from build123d import *

# Parameters (mm, degrees)
BOSS_EXTRUDE1_DEPTH = 120
SKETCH3_W           = 120
SKETCH3_H           = 10
BOSS_EXTRUDE2_DEPTH = 50
SKETCH11_R          = 13
CUT_EXTRUDE3_DEPTH  = 120
SKETCH7_R           = 1.825
SKETCH7_R_2         = 2
CUT_EXTRUDE6_DEPTH  = 5
CUT_EXTRUDE12_DEPTH = 4
SKETCH10_R          = 13
CUT_EXTRUDE13_DEPTH = 116
SKETCH8_R           = 1.825
SKETCH8_R_2         = 2
CUT_EXTRUDE14_DEPTH = 5
SKETCH13_R          = 13
CUT_EXTRUDE17_DEPTH = 120
SKETCH17_R          = 13
CUT_EXTRUDE18_DEPTH = 6
SKETCH18_R          = 1.75
CUT_EXTRUDE19_DEPTH = 6
FILLET1_R           = 3
FILLET2_R           = 3
CHAMFER1_SIZE       = 3
SKETCH19_W          = 15
SKETCH19_H          = 15
CUT_EXTRUDE20_DEPTH = 115
SKETCH20_R          = 5
CUT_EXTRUDE21_DEPTH = 5
FILLET3_R           = 3
SKETCH21_W          = 15
SKETCH21_H          = 15
CUT_EXTRUDE22_DEPTH = 5
SKETCH22_R          = 5
CUT_EXTRUDE23_DEPTH = 5
FILLET4_R           = 3
CUT_EXTRUDE24_START = -5
SKETCH23_R          = 1.825
SKETCH23_R_2        = 2
CUT_EXTRUDE24_DEPTH = 5
CUT_EXTRUDE25_START = -5
SKETCH24_R          = 1.825
SKETCH24_R_2        = 2
CUT_EXTRUDE25_DEPTH = 5
SKETCH26_R          = 1.825
SKETCH26_R_2        = 2
CUT_EXTRUDE26_DEPTH = 5


with BuildPart() as part:
    # Sketch1 → Boss-Extrude1 (new body)
    with BuildSketch(Plane(origin=(0, 0, 0), x_dir=(1, 0, 0), z_dir=(0, 1, 0))):
        Polygon((-60, 60), (-60, -60), (60, -60), (60, 60), (0, 60), align=None)
    extrude(amount=BOSS_EXTRUDE1_DEPTH)

    # Sketch3 → Boss-Extrude2 (add)
    with BuildSketch(Plane(origin=(60, 0, 0), x_dir=(0, 0, -1), z_dir=(1, 0, 0))):
        with Locations((0, 5)):
            Rectangle(SKETCH3_W, SKETCH3_H)
    extrude(amount=BOSS_EXTRUDE2_DEPTH)

    # Sketch11 → Cut-Extrude3 (cut)
    with BuildSketch(Plane.XY.offset(60)):
        with Locations((0, 60)):
            Circle(SKETCH11_R)
    extrude(amount=-CUT_EXTRUDE3_DEPTH, mode=Mode.SUBTRACT)

    # Sketch7 → Cut-Extrude6 (cut)
    with BuildSketch(Plane.ZY.offset(60)):
        with Locations((0, 76)):
            Circle(SKETCH7_R)
        with Locations((13.856406461, 52)):
            Circle(SKETCH7_R)
        with Locations((-13.856406461, 52)):
            Circle(SKETCH7_R)
        with Locations((-38.183766184, 98.183766184)):
            Circle(SKETCH7_R_2)
        with Locations((38.183766184, 98.183766184)):
            Circle(SKETCH7_R_2)
        with Locations((38.183766184, 21.816233816)):
            Circle(SKETCH7_R_2)
        with Locations((-38.183766184, 21.816233816)):
            Circle(SKETCH7_R_2)
    extrude(amount=-CUT_EXTRUDE6_DEPTH, mode=Mode.SUBTRACT)

    # Sketch4 → Cut-Extrude12 (cut)
    with BuildSketch(Plane.XZ):
        Polygon((16, 16), (110, 16), (110, -16), (16, -16), (16, -60), (-16, -60), (-16, -16), (-60, -16), (-60, 16), (-16, 16), (-16, 60), (16, 60), align=None)
    extrude(amount=-CUT_EXTRUDE12_DEPTH, mode=Mode.SUBTRACT)

    # Sketch10 → Cut-Extrude13 (cut)
    with BuildSketch(Plane(origin=(0, 120, 0), x_dir=(1, 0, 0), z_dir=(0, 1, 0))):
        with Locations(Location((0, 0, 0), (0, 0, 270))):
            Circle(SKETCH10_R)
    extrude(amount=-CUT_EXTRUDE13_DEPTH, mode=Mode.SUBTRACT)

    # Sketch8 → Cut-Extrude14 (cut)
    with BuildSketch(Plane(origin=(0, 0, -60), x_dir=(-1, 0, 0), z_dir=(0, 0, -1))):
        with Locations((0, 76)):
            Circle(SKETCH8_R)
        with Locations((13.856406461, 52)):
            Circle(SKETCH8_R)
        with Locations((-13.856406461, 52)):
            Circle(SKETCH8_R)
        with Locations((-38.183766184, 98.183766184)):
            Circle(SKETCH8_R_2)
        with Locations((38.183766184, 98.183766184)):
            Circle(SKETCH8_R_2)
        with Locations((38.183766184, 21.816233816)):
            Circle(SKETCH8_R_2)
        with Locations((-38.183766184, 21.816233816)):
            Circle(SKETCH8_R_2)
    extrude(amount=-CUT_EXTRUDE14_DEPTH, mode=Mode.SUBTRACT)

    # Sketch13 → Cut-Extrude17 (cut)
    with BuildSketch(Plane(origin=(60, 0, 0), x_dir=(0, 0, -1), z_dir=(1, 0, 0))):
        with Locations((0, 60)):
            Circle(SKETCH13_R)
    extrude(amount=-CUT_EXTRUDE17_DEPTH, mode=Mode.SUBTRACT)

    # Sketch17 → Cut-Extrude18 (cut)
    with BuildSketch(Plane(origin=(0, 10, 0), x_dir=(1, 0, 0), z_dir=(0, 1, 0))):
        with Locations(Location((85, 0, 0), (0, 0, 270))):
            Circle(SKETCH17_R)
    extrude(amount=-CUT_EXTRUDE18_DEPTH, mode=Mode.SUBTRACT)

    # Sketch18 → Cut-Extrude19 (cut)
    with BuildSketch(Plane(origin=(0, 10, 0), x_dir=(1, 0, 0), z_dir=(0, 1, 0))):
        with Locations(Location((93, 13.856406461, 0), (0, 0, 270))):
            Circle(SKETCH18_R)
        with Locations(Location((69, 0, 0), (0, 0, 270))):
            Circle(SKETCH18_R)
        with Locations(Location((93, -13.856406461, 0), (0, 0, 270))):
            Circle(SKETCH18_R)
    extrude(amount=-CUT_EXTRUDE19_DEPTH, mode=Mode.SUBTRACT)

    # Fillet1
    fillet1_edges = [part.edges().sort_by_distance(p)[0] for p in [
        (16, 2, -16),
        (-16, 2, -16),
        (-16, 2, 16),
        (16, 2, 16),
    ]]
    fillet(fillet1_edges, radius=FILLET1_R)

    # Fillet2
    fillet2_edges = [part.edges().sort_by_distance(p)[0] for p in [
        (0, 4, -13),
    ]]
    fillet(fillet2_edges, radius=FILLET2_R)

    # Chamfer1
    chamfer1_edges = [part.edges().sort_by_distance(p)[0] for p in [
        (0, 4, 60),
        (110, 4, 0),
        (0, 4, -60),
        (-60, 4, 0),
    ]]
    chamfer(chamfer1_edges, length=CHAMFER1_SIZE)

    # Sketch19 → Cut-Extrude20 (cut)
    with BuildSketch(Plane(origin=(0, 120, 0), x_dir=(1, 0, 0), z_dir=(0, 1, 0))):
        with Locations((-52.5, 52.5)):
            Rectangle(SKETCH19_W, SKETCH19_H)
        with Locations((-52.5, -52.5)):
            Rectangle(SKETCH19_W, SKETCH19_H)
    extrude(amount=-CUT_EXTRUDE20_DEPTH, mode=Mode.SUBTRACT)

    # Sketch20 → Cut-Extrude21 (cut)
    with BuildSketch(Plane(origin=(0, 5, 0), x_dir=(1, 0, 0), z_dir=(0, 1, 0))):
        with Locations(Location((-52.5, 52.5, 0), (0, 0, 270))):
            Circle(SKETCH20_R)
        with Locations(Location((-52.5, -52.5, 0), (0, 0, 270))):
            Circle(SKETCH20_R)
    extrude(amount=-CUT_EXTRUDE21_DEPTH, mode=Mode.SUBTRACT)

    # Fillet3
    fillet3_edges = [part.edges().sort_by_distance(p)[0] for p in [
        (-45, 62.5, -45),
        (-45, 62.5, 45),
    ]]
    fillet(fillet3_edges, radius=FILLET3_R)

    # Sketch21 → Cut-Extrude22 (cut)
    with BuildSketch(Plane(origin=(0, 10, 0), x_dir=(1, 0, 0), z_dir=(0, 1, 0))):
        with Locations((102.5, -52.5)):
            Rectangle(SKETCH21_W, SKETCH21_H)
        with Locations((102.5, 52.5)):
            Rectangle(SKETCH21_W, SKETCH21_H)
    extrude(amount=-CUT_EXTRUDE22_DEPTH, mode=Mode.SUBTRACT)

    # Sketch22 → Cut-Extrude23 (cut)
    with BuildSketch(Plane(origin=(0, 5, 0), x_dir=(1, 0, 0), z_dir=(0, 1, 0))):
        with Locations(Location((102.5, 52.5, 0), (0, 0, 270))):
            Circle(SKETCH22_R)
        with Locations(Location((102.5, -52.5, 0), (0, 0, 270))):
            Circle(SKETCH22_R)
    extrude(amount=-CUT_EXTRUDE23_DEPTH, mode=Mode.SUBTRACT)

    # Fillet4
    fillet4_edges = [part.edges().sort_by_distance(p)[0] for p in [
        (95, 7.5, 45),
        (95, 7.5, -45),
    ]]
    fillet(fillet4_edges, radius=FILLET4_R)

    # Sketch23 → Cut-Extrude24 (cut)
    with BuildSketch(Plane.XY.offset(60).offset(CUT_EXTRUDE24_START)):
        with Locations((0.077859326, 75.922140674)):
            Circle(SKETCH23_R)
        with Locations((13.934265787, 51.922140674)):
            Circle(SKETCH23_R)
        with Locations((-13.778547134, 51.922140674)):
            Circle(SKETCH23_R)
        with Locations(Location((-38.183766184, 98.183766184, 0), (0, 0, 180))):
            Circle(SKETCH23_R_2)
        with Locations(Location((38.183766184, 98.183766184, 0), (0, 0, 180))):
            Circle(SKETCH23_R_2)
        with Locations(Location((38.183766184, 21.816233816, 0), (0, 0, 180))):
            Circle(SKETCH23_R_2)
        with Locations(Location((-38.183766184, 21.816233816, 0), (0, 0, 180))):
            Circle(SKETCH23_R_2)
    extrude(amount=CUT_EXTRUDE24_DEPTH, mode=Mode.SUBTRACT)

    # Sketch24 → Cut-Extrude25 (cut)
    with BuildSketch(Plane(origin=(60, 0, 0), x_dir=(0, 0, -1), z_dir=(1, 0, 0)).offset(CUT_EXTRUDE25_START)):
        with Locations(Location((0, 76, 0), (0, 0, 180))):
            Circle(SKETCH24_R)
        with Locations(Location((13.856406461, 52, 0), (0, 0, 180))):
            Circle(SKETCH24_R)
        with Locations(Location((-13.856406461, 52, 0), (0, 0, 180))):
            Circle(SKETCH24_R)
        with Locations(Location((-38.183766184, 98.183766184, 0), (0, 0, 180))):
            Circle(SKETCH24_R_2)
        with Locations(Location((38.183766184, 98.183766184, 0), (0, 0, 180))):
            Circle(SKETCH24_R_2)
        with Locations(Location((38.183766184, 21.816233816, 0), (0, 0, 180))):
            Circle(SKETCH24_R_2)
        with Locations(Location((-38.183766184, 21.816233816, 0), (0, 0, 180))):
            Circle(SKETCH24_R_2)
    extrude(amount=CUT_EXTRUDE25_DEPTH, mode=Mode.SUBTRACT)

    # Sketch26 → Cut-Extrude26 (cut)
    with BuildSketch(Plane(origin=(0, 120, 0), x_dir=(1, 0, 0), z_dir=(0, 1, 0))):
        with Locations(Location((0, 16, 0), (0, 0, 270))):
            Circle(SKETCH26_R)
        with Locations(Location((13.856406461, -8, 0), (0, 0, 270))):
            Circle(SKETCH26_R)
        with Locations(Location((-13.856406461, -8, 0), (0, 0, 270))):
            Circle(SKETCH26_R)
        with Locations(Location((-38.183766184, 38.183766184, 0), (0, 0, 270))):
            Circle(SKETCH26_R_2)
        with Locations(Location((38.183766184, 38.183766184, 0), (0, 0, 270))):
            Circle(SKETCH26_R_2)
        with Locations(Location((38.183766184, -38.183766184, 0), (0, 0, 270))):
            Circle(SKETCH26_R_2)
        with Locations(Location((-38.183766184, -38.183766184, 0), (0, 0, 270))):
            Circle(SKETCH26_R_2)
    extrude(amount=-CUT_EXTRUDE26_DEPTH, mode=Mode.SUBTRACT)


solid = part.part
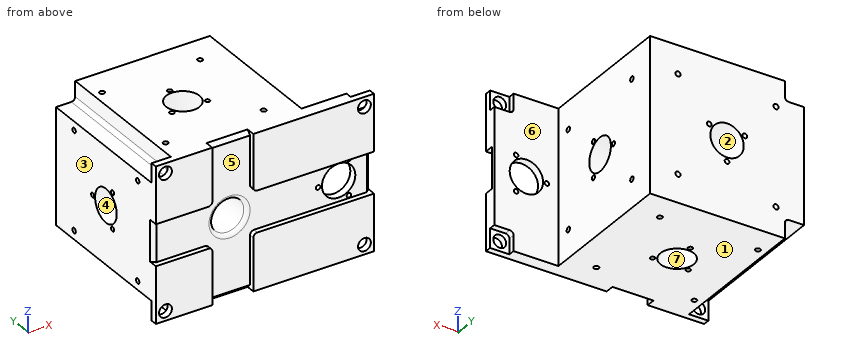
Build history of the part. All positions in model axes, mm. Face numbers are marked on the shaded views. A direction names the side the tool comes from. Round coordinates to 2 decimals unless told otherwise and drop trailing zeros. Write each loop counter-clockwise with the first axis right and the second up, starting at its lowest first coordinate (ties: lowest second). Pieces come first, ordered by that corner, then holes. Notation, with made-up numbers: M 30,84.5 L 39,84.5 A16 ccw 39,110.5 Z; hole C 78,30.5 d11. An arc over 180 degrees is marked long. Use CSV: the item, a comma, the result in double quotes.
1. Two-plate mould, pull along Z, no slides. Class the marked faces 1, 2, 3 and 4: +Z half, -Z half, draft (parallel to the pull), parting line (faces both ways), or undercut.
Reply:
face 1,"-Z half"
face 2,"undercut"
face 3,"draft"
face 4,"undercut"
2. Saw through at C-C (y = 41). Give the cut face in (x, z), plus the area to 3 significant figures.
Reply:
outline,"M -60,-45 L -48,-45 A3 cw -45,-48 L -45,-60 L 60,-60 L 60,60 L -45,60 L -45,48 A3 cw -48,45 L -60,45 Z; hole C 0,0 d26"
area,"13,400 mm²"
3. Saw through at A-A (x = 102.5). Give the cut face in (y, z).
Reply:
outline,"M 0,-60 L 5,-60 L 5,-57.5 L 0,-57.5 Z; M 0,-47.5 L 5,-47.5 L 5,-45 L 10,-45 L 10,45 L 5,45 L 5,47.5 L 0,47.5 L 0,16 L 4,16 L 4,-16 L 0,-16 Z; M 0,57.5 L 5,57.5 L 5,60 L 0,60 Z"
4. Wall check: probe 1 along X at (y, z) = (117.95, -16) (3 decimals); probe 2 along Z at (x, y) = (69, 7). Give the ranges that are in metal, low to high. Write a range as from..to.
Reply:
probe 1,"x = -60..-1.825, 1.825..60"
probe 2,"z = -60..-1.75, 1.75..60"
5. Saw through at D-D (z = 30). Give the cut face in (x, y), plus the area to 3 significant figures.
Reply:
outline,"M -60,0 L -16,0 L -16,4 L 16,4 L 16,0 L 110,0 L 110,10 L 60,10 L 60,120 L -60,120 Z; hole C 0,60 d26"
area,"14,200 mm²"
6. Tool access for the marked faces 5, 6 and 7: list every direction of +Z, -Z, +X, -X, +Y, -Y with a clear straight run to the whole face (end or side of a thin tool).
Reply:
face 5,"-Y"
face 6,"+Z, -Z, +X, +Y"
face 7,"+Z, -Z"
7. Saw through at B-B (z = 52.5). Give the cut face in (x, y).
Reply:
outline,"M -60,0 L -57.5,0 L -57.5,5 L -60,5 Z; M -47.5,0 L -16,0 L -16,4 L 16,4 L 16,0 L 97.5,0 L 97.5,5 L 95,5 L 95,10 L 60,10 L 60,120 L -45,120 L -45,5 L -47.5,5 Z; M 107.5,0 L 110,0 L 110,5 L 107.5,5 Z; hole C 0,60 d26"
8. Flat gauge pins, fed straight in: pin 1 (3 mm diameter, centred on x = 38.18, z = 38.18, fed in from +Y); pin 2 (3 mm diameter, centred on y = 52, z = -13.86, fed in from +X); pin 3 (1.5 mm diameter, centred on x = -4.5, z = -35.5, fed in from -Y). Where does each tip first touch, or does it go through?
Reply:
pin 1,"stops at y = 115"
pin 2,"stops at x = 55"
pin 3,"stops at y = 4"
